from build123d import *

# Parameters (mm, degrees)
F0_W     = 76.2
F0_H     = 38.1
F0_W_2   = 6.35
F0_H_2   = 6.35
F0_W_3   = 9.525
F0_H_3   = 9.525
F0_W_4   = 12.7
F0_H_4   = 12.7
F0_R     = 4.7625
F0_R_2   = 3.175
F0_R_3   = 6.35
F1_DEPTH = 1.5875
F2_R     = 6.35
F3_SIZE  = 6.35


with BuildPart() as f1:
    # F0 (on Front) → F1 (new body, symmetric)
    with BuildSketch(Plane.XZ):
        Rectangle(F0_W, F0_H)
        with Locations((-28.530458, -11.846916)):
            Rectangle(F0_W_2, F0_H_2, mode=Mode.SUBTRACT)
        with Locations((-14.919388, -11.971785)):
            Rectangle(F0_W_3, F0_H_3, mode=Mode.SUBTRACT)
        with Locations((20.656448, -8.97043)):
            Rectangle(F0_W_4, F0_H_4, mode=Mode.SUBTRACT)
        with Locations((-18.023899, 6.521787)):
            Circle(F0_R, mode=Mode.SUBTRACT)
        with Locations((-28.73469, 10.823162)):
            Circle(F0_R_2, mode=Mode.SUBTRACT)
        Polygon((-10.998523, 0), (-5.499261, 9.525), (5.499261, 9.525), (10.998523, 0), (5.499261, -9.525), (-5.499261, -9.525), align=None, mode=Mode.SUBTRACT)
        with Locations((23.2064, 8.776863)):
            Circle(F0_R_3, mode=Mode.SUBTRACT)
    extrude(amount=F1_DEPTH, both=True)

    # F2
    f2_edges = [f1.edges().sort_by_distance(p)[0] for p in [
        (-38.1, 0, 19.05),
        (-38.1, 0, -19.05),
    ]]
    fillet(f2_edges, radius=F2_R)

    # F3
    f3_edges = [f1.edges().sort_by_distance(p)[0] for p in [
        (38.1, 0, 19.05),
        (38.1, 0, -19.05),
    ]]
    chamfer(f3_edges, length=F3_SIZE)


solid = f1.part
For this review, take the finished solid that the model builds, in its own axes (mm). A direction names the side the tool comes from. Coordinates: 2 decimals unless noted, no trailing zeros. Order: outer loops, then holes, each group sorted by start corner. A loop starts at its lowest first (then second) coordinate and runs counter-clockwise, first axis right, second up. Notation, with made-up numbers: (77, 47.25) -> (92, 47.25) arc R18 cw to (92, 52.25) -> close; hole circle Ø7 at (46, 5). An arc over 180 degrees is marked (long way). Return JSON: item names as keys, results as strings.
1. For line 1 (Z direction, x = -3, y = -1.35) (3 decimals); line 2 (Z direction, x = -14, y = 0.5), list the stretches that pass through material, from the lowest coordinate up. Write a range as from..to.
Answer block:
{"line 1": "-19.05..-9.525, 9.525..19.05", "line 2": "-19.05..-16.73, -7.21..3.97, 9.07..19.05"}
2. Machinability: for faces 1 (the cylindrical face through (-36.29, -0.02, -17.14)), 2 (the flat face through (0, 0, 9.525)), which of the approach directions +Z, -Z, +X, -X, +Y, -Y give a long, thin tool a straight path to every point of the face, cutting with its end or side? Answer none if there is none.
Answer block:
{"face 1": "-Z, -X, +Y, -Y", "face 2": "+Y, -Y"}
3. For pin 1 Ø10 at (x, z) = (24.5, -11.5) entering from -Y; pin 2 Ø5 at (x, z) = (-28.73, 10.82) entering from +Y, all flat-tipped, find the tip position at first contact; note any pin that passes through.
Answer block:
{"pin 1": "y = -1.59", "pin 2": "through"}
4. The part is to be moulded in two halves that separate along X. For faces 3 (the flat face through (38.1, 0, 0)), 4 (the flat face through (-25.355, 0, -12)), 5 (the flat face through (-38.1, 0, 0)), say which applies: +X half, -X half, draft (parallel to the pull), parting line (faces both ways), or undercut.
Answer block:
{"face 3": "+X half", "face 4": "undercut", "face 5": "-X half"}
5. We need section C-C on y = -0.7. State how many separate pieces and enclosed holes the cut face has, and give its area (3 significant figures).
Answer block:
{"separate pieces": "1", "enclosed holes": "7", "area": "2,010 mm²"}
6. We need section B-B on z = -6. Write out the cut boundary in (x, y).
Answer block:
{"outline": "(-38.1, -1.59) -> (-7.53, -1.59) -> (-7.53, 1.59) -> (-38.1, 1.59) -> close; (7.53, -1.59) -> (14.31, -1.59) -> (14.31, 1.59) -> (7.53, 1.59) -> close; (27.01, -1.59) -> (38.1, -1.59) -> (38.1, 1.59) -> (27.01, 1.59) -> close"}
7. We need section D-D on x = -14.5. Write out the cut boundary in (y, z), and give its area (3 significant figures).
Answer block:
{"outline": "(-1.59, -19.05) -> (1.59, -19.05) -> (1.59, -16.73) -> (-1.59, -16.73) -> close; (-1.59, -7.21) -> (1.59, -7.21) -> (1.59, 3.32) -> (-1.59, 3.32) -> close; (-1.59, 9.73) -> (1.59, 9.73) -> (1.59, 19.05) -> (-1.59, 19.05) -> close", "area": "70.4 mm²"}
